Verification items for the finished model (mm, model axes). A direction names the side the tool comes from. Round coordinates to 2 decimals unless told otherwise and drop trailing zeros. Write each loop counter-clockwise with the first axis right and the second up, starting at its lowest first coordinate (ties: lowest second). Pieces come first, ordered by that corner, then holes. Notation, with made-up numbers: (-12.75, -18.5) -> (3.25, -18.5) arc R7 cw to (3.25, -8.5) -> close; hole circle Ø1 at (-2.75, -12.75). An arc over 180 degrees is marked (long way). Use CSV: the item, a comma, the result in double quotes.
```python
from build123d import *

# Parameters (mm, degrees)
BOSS_1_DEPTH  = 6
S_CYL2_R      = 12.5
BOSS_2_DEPTH  = 2
S_HOLE3_R     = 3.5
HOLE_3_DEPTH  = 8.2
S_HOLE4_R     = 1.7
HOLE_4_DEPTH  = 8.2
S_HOLE5_R     = 1.7
HOLE_5_DEPTH  = 8.2
S_HOLE6_R     = 1.7
HOLE_6_DEPTH  = 8.2
S_HOLE7_R     = 1.7
HOLE_7_DEPTH  = 8.2
S_HOLE8_R     = 3.2
HOLE_8_DEPTH  = 5.1
S_HOLE9_R     = 3.2
HOLE_9_DEPTH  = 5.1
S_HOLE10_R    = 3.2
HOLE_10_DEPTH = 5.1
S_HOLE11_R    = 3.2
HOLE_11_DEPTH = 5.1


with BuildPart() as part:
    # S_prism1 → Boss_1 (new body)
    with BuildSketch(Plane(origin=(0, 0, 0), x_dir=(1, 0, 0), z_dir=(0, 1, 0))):
        with BuildLine():
            Line((-1, -16), (1.6805, -16))
            ThreePointArc((1.6805, -16), (12.745771818, -11.556826983), (17.6654, -0.695))
            Line((17.6654, -0.695), (19, 30))
            Line((19, 30), (13.7468, 108.7982))
            ThreePointArc((13.7468, 108.7982), (9.971633889, 116.762968295), (1.7734, 120))
            Line((1.7734, 120), (0.2266, 120))
            ThreePointArc((0.2266, 120), (-7.971633889, 116.762968295), (-11.7468, 108.7982))
            Line((-11.7468, 108.7982), (-17, 30))
            Line((-17, 30), (-17, 0))
            ThreePointArc((-17, 0), (-12.3137, -11.3137), (-1, -16))
        make_face()
    extrude(amount=BOSS_1_DEPTH)

    # S_cyl2 → Boss_2 (add)
    with BuildSketch(Plane(origin=(0, 6, 0), x_dir=(1, 0, 0), z_dir=(0, 1, 0))):
        with Locations(Location((0, 0, 0), (0, 0, 270))):
            Circle(S_CYL2_R)
    extrude(amount=BOSS_2_DEPTH)

    # S_hole3 → Hole_3 (cut)
    with BuildSketch(Plane(origin=(0, -0.1, 0), x_dir=(1, 0, 0), z_dir=(0, 1, 0))):
        with Locations(Location((0, 0, 0), (0, 0, 270))):
            Circle(S_HOLE3_R)
    extrude(amount=HOLE_3_DEPTH, mode=Mode.SUBTRACT)

    # S_hole4 → Hole_4 (cut)
    with BuildSketch(Plane(origin=(0, -0.1, 0), x_dir=(1, 0, 0), z_dir=(0, 1, 0))):
        with Locations(Location((7, 0, 0), (0, 0, 270))):
            Circle(S_HOLE4_R)
    extrude(amount=HOLE_4_DEPTH, mode=Mode.SUBTRACT)

    # S_hole5 → Hole_5 (cut)
    with BuildSketch(Plane(origin=(0, -0.1, 0), x_dir=(1, 0, 0), z_dir=(0, 1, 0))):
        with Locations(Location((0, -7, 0), (0, 0, 270))):
            Circle(S_HOLE5_R)
    extrude(amount=HOLE_5_DEPTH, mode=Mode.SUBTRACT)

    # S_hole6 → Hole_6 (cut)
    with BuildSketch(Plane(origin=(0, -0.1, 0), x_dir=(1, 0, 0), z_dir=(0, 1, 0))):
        with Locations(Location((-7, 0, 0), (0, 0, 270))):
            Circle(S_HOLE6_R)
    extrude(amount=HOLE_6_DEPTH, mode=Mode.SUBTRACT)

    # S_hole7 → Hole_7 (cut)
    with BuildSketch(Plane(origin=(0, -0.1, 0), x_dir=(1, 0, 0), z_dir=(0, 1, 0))):
        with Locations(Location((0, 7, 0), (0, 0, 270))):
            Circle(S_HOLE7_R)
    extrude(amount=HOLE_7_DEPTH, mode=Mode.SUBTRACT)

    # S_hole8 → Hole_8 (cut)
    with BuildSketch(Plane(origin=(0, 3, 0), x_dir=(1, 0, 0), z_dir=(0, 1, 0))):
        with Locations(Location((7, 0, 0), (0, 0, 270))):
            Circle(S_HOLE8_R)
    extrude(amount=HOLE_8_DEPTH, mode=Mode.SUBTRACT)

    # S_hole9 → Hole_9 (cut)
    with BuildSketch(Plane(origin=(0, 3, 0), x_dir=(1, 0, 0), z_dir=(0, 1, 0))):
        with Locations(Location((0, -7, 0), (0, 0, 270))):
            Circle(S_HOLE9_R)
    extrude(amount=HOLE_9_DEPTH, mode=Mode.SUBTRACT)

    # S_hole10 → Hole_10 (cut)
    with BuildSketch(Plane(origin=(0, 3, 0), x_dir=(1, 0, 0), z_dir=(0, 1, 0))):
        with Locations(Location((-7, 0, 0), (0, 0, 270))):
            Circle(S_HOLE10_R)
    extrude(amount=HOLE_10_DEPTH, mode=Mode.SUBTRACT)

    # S_hole11 → Hole_11 (cut)
    with BuildSketch(Plane(origin=(0, 3, 0), x_dir=(1, 0, 0), z_dir=(0, 1, 0))):
        with Locations(Location((0, 7, 0), (0, 0, 270))):
            Circle(S_HOLE11_R)
    extrude(amount=HOLE_11_DEPTH, mode=Mode.SUBTRACT)


solid = part.part
```
Q1. Mould release check, pull along X, two halves, no side actions. Record for faces 3 (the flat face through (5.6, 3, 1.4)), 4 (the flat face through (-14.337, 2.958, -69.951)), 5 (the flat face through (16.41, 2.96, -68.85)): released by +X, released by -X, zero draft, split by the parting line, or undercut.
Filled in:
face 3,"undercut"
face 4,"released by -X"
face 5,"released by +X"
Q2. Section check A-A (y = 4.5). Record the cut outline in (x, z) (1 decimal), plus the area to 3 significant figures.
Filled in:
outline,"(-17, -30) -> (-11.7, -108.8) arc R12 ccw to (0.2, -120) -> (1.8, -120) arc R12 ccw to (13.7, -108.8) -> (19, -30) -> (17.7, 0.7) arc R16 ccw to (1.7, 16) -> (-1, 16) arc R16 ccw to (-17, 0) -> close; hole circle Ø6.4 at (-7, 0); hole circle Ø7 at (0, 0); hole circle Ø6.4 at (0, -7); hole circle Ø6.4 at (0, 7); hole circle Ø6.4 at (7, 0)"
area,"3,990 mm²"
Q3. Section check D-D (z = -36). Record the cut outline in (x, y).
Filled in:
outline,"(-16.6, 0) -> (18.6, 0) -> (18.6, 6) -> (-16.6, 6) -> close"
Q4. Access from +Z, -Z, +X, -X, +Y, -Y to the whole of each face (thin tool, end or side, straight path). Record for faces 1 (the cylindrical face through (7.961, 5.465, 3.052)), 2 (the cylindrical face through (-7.88, 2.96, -116.85)).
Filled in:
face 1,"+Y"
face 2,"-Z, -X, +Y, -Y"
Q5. Section check B-B (x = 7). Record the cut outline in (y, z), plus the area to 3 significant figures.
Filled in:
outline,"(0, -118.8) -> (6, -118.8) -> (6, -10.36) -> (8, -10.36) -> (8, -3.2) -> (3, -3.2) -> (3, -1.7) -> (0, -1.7) -> close; (0, 1.7) -> (3, 1.7) -> (3, 3.2) -> (8, 3.2) -> (8, 10.36) -> (6, 10.36) -> (6, 15.09) -> (0, 15.09) -> close"
area,"803 mm²"
Q6. Material ranges on L1, parallel to Z at x = 0, y = 1.85; L2, parallel to Z at x = 0, y = 4.95; L3, parallel to X at y = 1, z = -109, recorded low to high.
Filled in:
L1,"-120 to -8.7, -5.3 to -3.5, 3.5 to 5.3, 8.7 to 16"
L2,"-120 to -10.2, -3.8 to -3.5, 3.5 to 3.8, 10.2 to 16"
L3,"-11.73 to 13.73"
Q7. Section check C-C (z = 7). Record the cut outline in (x, y).
Filled in:
outline,"(-15.39, 0) -> (-1.7, 0) -> (-1.7, 3) -> (-3.2, 3) -> (-3.2, 8) -> (-10.36, 8) -> (-10.36, 6) -> (-15.39, 6) -> close; (1.7, 0) -> (16.07, 0) -> (16.07, 6) -> (10.36, 6) -> (10.36, 8) -> (3.2, 8) -> (3.2, 3) -> (1.7, 3) -> close"
Q8. Go/stop test with flat-tipped pins: P1, Ø3, axis at x = -3, z = -15.5, coming from the +Y side; P2, Ø2, axis at x = -7, z = 0, coming from the -Y side; P3, Ø4.5, axis at x = 7, z = 0, coming from the +Y side. Record where each tip stops, or that it passes through.
Filled in:
P1,"y = 6"
P2,"through"
P3,"y = 3"
